Autodesk Inventor part; units mm, degrees
ref_plane "YZ Plane" through (0, 0, 0) normal (1, 0, 0) x (0, 1, 0)
ref_plane "XZ Plane" through (0, 0, 0) normal (0, 1, 0) x (-1, 0, 0)
ref_plane "XY Plane" through (0, 0, 0) normal (0, 0, 1) x (1, 0, 0)
sketch "Sketch1" plane through (0, 0, 0) normal (0, 0, 1) x (1, 0, 0)
  line L0 (0, 0) -> (140, 0)
  line L1 (140, 0) -> (140, 140)
  line L2 (140, 140) -> (0, 140)
  line L3 (0, 140) -> (0, 0)
  dimension "d0" = 140
  dimension "d1" = 140
extrude "Extrusion1" add sketch "Sketch1" along normal blind 5
fillet "Fillet1" radius 5 4 edges at (140, 140, 2.5) (140, 0, 2.5) (0, 140, 2.5) (0, 0, 2.5)
sketch "Sketch4" plane through (0, 0, 5) normal (0, 0, 1) x (1, 0, 0)
  line L0 (135, 140) -> (5, 140)
  line L1 (0, 135) -> (0, 5)
  line L2 (140, 5) -> (140, 135)
  line L3 (5, 0) -> (135, 0)
  point P0 (0, 0)
  point P1 (6, 134)
  point P2 (134, 134)
  point P3 (6, 6)
  point P4 (134, 6)
  dimension "d30" = 6
  dimension "d31" = 6
  dimension "d32" = 6
  dimension "d33" = 6
  dimension "d34" = 6
  dimension "d35" = 6
  dimension "d36" = 6
  dimension "d37" = 6
hole "Hole2" at (134, 134, 5) at (6, 6, 5) at (134, 6, 5) at (6, 134, 5) direction (0, 0, -1) diameter 4 depth 15
sketch "Sketch5" plane through (0, 0, 5) normal (0, 0, 1) x (1, 0, 0)
  line L0 (20, 130) -> (120, 130)
  line L1 (120, 130) -> (120, 125)
  line L2 (120, 125) -> (20, 125)
  line L3 (20, 125) -> (20, 130)
  line L4 (135, 140) -> (5, 140)
  line L5 (140, 5) -> (140, 135)
  line L6 (20, 15) -> (120, 15)
  line L7 (120, 15) -> (120, 10)
  line L8 (120, 10) -> (20, 10)
  line L9 (20, 10) -> (20, 15)
  line L10 (5, 0) -> (135, 0)
  line L11 (10, 120) -> (15, 120)
  line L12 (15, 120) -> (15, 20)
  line L13 (15, 20) -> (10, 20)
  line L14 (10, 20) -> (10, 120)
  line L15 (0, 135) -> (0, 5)
  line L16 (125, 120) -> (130, 120)
  line L17 (130, 120) -> (130, 20)
  line L18 (130, 20) -> (125, 20)
  line L19 (125, 20) -> (125, 120)
  point P0 (0, 0)
  dimension "d45" = 10
  dimension "d46" = 5
  dimension "d47" = 20
  dimension "d48" = 100
  dimension "d49" = 100
  dimension "d50" = 5
  dimension "d51" = 20
  dimension "d52" = 10
  dimension "d53" = 5
  dimension "d54" = 100
  dimension "d55" = 20
  dimension "d56" = 10
  dimension "d57" = 5
  dimension "d58" = 100
  dimension "d59" = 10
  dimension "d60" = 20
extrude "Extrusion4" cut sketch "Sketch5" against normal blind 10
properties part number "Led deksel niet hub"
Here's how the part is built. I have some questions about the finished solid (model axes, mm). A direction names the side the tool comes from. Give positions to 0.01 mm unless a question says otherwise; leave off trailing zeros. Order: outer loops, then holes, each group sorted by start corner. A loop starts at its lowest first (then second) coordinate and runs counter-clockwise, first axis right, second up. Notation, with made-up numbers: (31.25, -24) -> (35.25, -24) arc R25 cw to (35.25, -11) -> close; hole circle Ø9 at (-21.75, -34). An arc over 180 degrees is marked (long way). One line per item, written item: value. Start each with the question number.
1. We'd pull the mould along Y, two halves only. Please class faces 3 (the face through (69, 0, 2)), 4 (the face through (69, 71, 0)), 5 (the face through (127, 120, 3)), 6 (the face through (125, 69, 3)): released by +Y, released by -Y, zero draft, split by the parting line, or undercut.
2. Will this pin go through, and if not, where does the flat tip stop? pin 1 Ø2.5 at (y, z) = (11.5, 2.5) entering from -X.
3. Imagine slicing it at B-B, the plane z = 1.9. Count the separate pieces of the cut face and the enclosed holes in it, plus the area to 3 significant figures.
4. I need wall thicknesses on probe 1 along Y at (x, z) = (80, 1.45); probe 2 along X at (y, z) = (134, 3.6). Which ranges of each line are inside material? Lowest first, please. Write a range as from..to.
5. Imagine slicing it at A-A, the plane x = 64.5. List the corners of the cut face in (y, z) for me, plus the area to 3 significant figures.
6. For faces 1 (the face through (130, 71, 3)), 2 (the face through (69, 71, 5)), which set-ups out of +Z, -Z, +X, -X, +Y, -Y let a thin tool reach every point of the face, with its end or its side?
Values follow:
1. face 3: released by -Y
1. face 4: zero draft
1. face 5: undercut
1. face 6: undercut
2. pin 1: stops at x = 0
3. separate pieces: 1
3. enclosed holes: 8
3. area: 17,500 mm2
4. probe 1: y = 0..10, 15..125, 130..140
4. probe 2: x = 0..4, 8..132, 136..140
5. outline: (0, 0) -> (10, 0) -> (10, 5) -> (0, 5) -> close; (15, 0) -> (125, 0) -> (125, 5) -> (15, 5) -> close; (130, 0) -> (140, 0) -> (140, 5) -> (130, 5) -> close
5. area: 650 mm2
6. face 1: +Z, -Z
6. face 2: +Z, +X, -X, +Y, -Y
